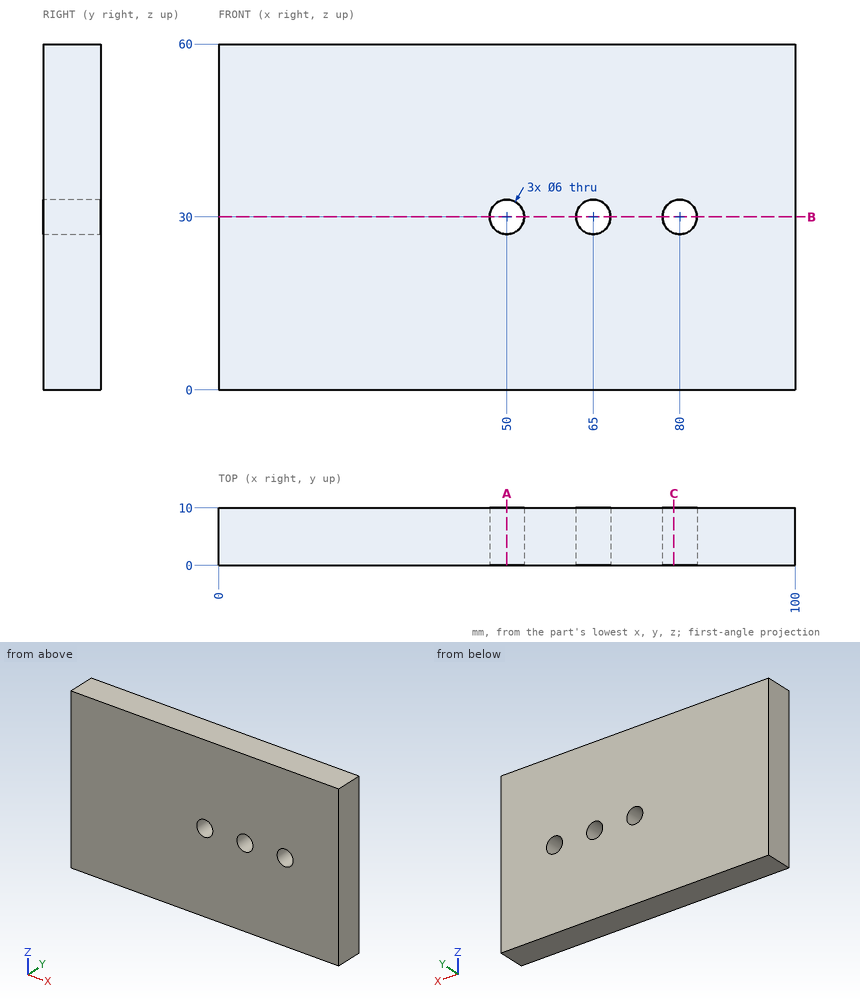
Could you check a few things on this drawing? It's one solid part, dimensions in mm from its lowest x, y, z. Give positions to 0.01 mm unless a question says otherwise; leave off trailing zeros. Loops run counter-clockwise (first coordinate to the right, second up) from the corner with the lowest first, then second, coordinate; pieces in that order, holes last. Notation, with made-up numbers: (15.25, 32) -> (33.25, 32) arc R17 cw to (33.25, 52) -> close; hole circle Ø11 at (54, 14.5). An arc over 180 degrees is marked (long way). Use one line per item in the form item = value. Start each with the question number.
1) For P1, Ø10, axis at x = 57, z = 12, coming from the -Y side, with a flat end and sliding along its axis, tell me the tip position at first contact or that it passes through.
2) Imagine slicing it at A-A (x = 50). Please give me the cut outline in (y, z).
3) Please list where these lines run through material, in increasing order: line 1 along X through (y, z) = (5.25, 30); line 2 along Z through (x, y) = (50, 4).
4) Imagine slicing it at B-B (z = 30). Please give me the cut outline in (x, y).
5) Imagine slicing it at C-C (x = 79). Please give me the cut outline in (y, z).
Check values:
q1.P1 = 0
q2.outline = (0, 0) -> (10, 0) -> (10, 27) -> (0, 27) -> close; (0, 33) -> (10, 33) -> (10, 60) -> (0, 60) -> close
q3.line_1 = 0 to 47, 53 to 62, 68 to 77, 83 to 100
q3.line_2 = 0 to 27, 33 to 60
q4.outline = (0, 0) -> (47, 0) -> (47, 10) -> (0, 10) -> close; (53, 0) -> (62, 0) -> (62, 10) -> (53, 10) -> close; (68, 0) -> (77, 0) -> (77, 10) -> (68, 10) -> close; (83, 0) -> (100, 0) -> (100, 10) -> (83, 10) -> close
q5.outline = (0, 0) -> (10, 0) -> (10, 27.17) -> (0, 27.17) -> close; (0, 32.83) -> (10, 32.83) -> (10, 60) -> (0, 60) -> close
